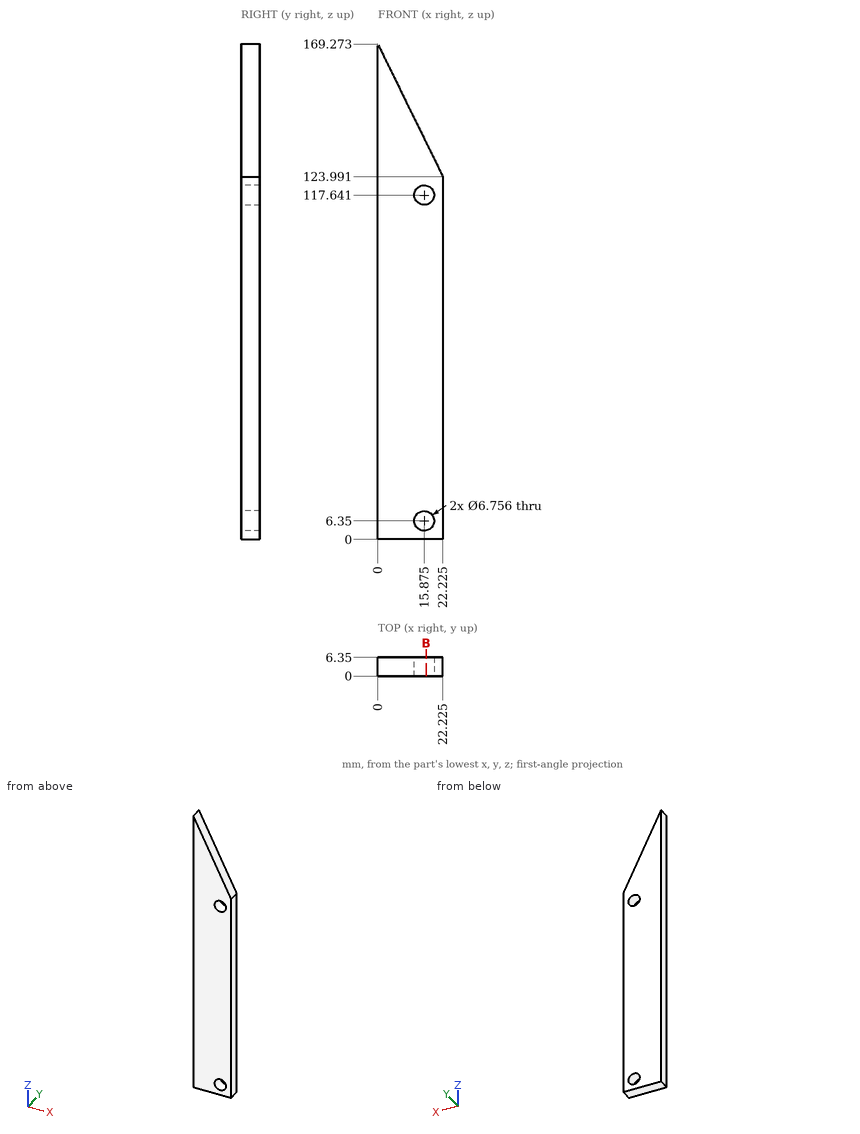
For this review, use the dimensioned drawing (mm, ordinates from the lowest corner) and the shaded views. Give positions to 0.01 mm unless a question says otherwise; leave off trailing zeros. Write each question's results on one line, items separated by ' | '.
(1) Take a section at B-B (x = 16.5). State how many separate pieces and enclosed holes the cut face has, then the cut area to 3 significant figures.
Conclusion:
separate pieces: 3 | enclosed holes: 0 | area: 777 mm^2
(2) For pin 1 Ø4 at (x, z) = (15.875, 6.35) entering from +Y, flat-tipped, find the tip position at first contact; note if it passes through.
Conclusion:
pin 1: through
(3) For line 1 along Z through (x, y) = (15.25, 5.75) (1 decimal); line 2 along Z through (x, y) = (13.75, 4) (1 decimal); line 3 along X through (y, z) = (2, 134), list the stretches that pass through material, from the lowest coordinate up.
Conclusion:
line 1: 0 to 3, 9.7 to 114.3, 121 to 138.2 | line 2: 0 to 3.7, 9 to 115, 120.3 to 141.3 | line 3: 0 to 17.31
